from build123d import *

# Parameters (mm, degrees)
SKETCH1_W           = 240
SKETCH1_H           = 148
SKETCH1_W_2         = 235
SKETCH1_H_2         = 143
BOSS_EXTRUDE1_DEPTH = 1.2


with BuildPart() as part:
    # Sketch1 → Boss-Extrude1 (new body)
    with BuildSketch(Plane.XY):
        Rectangle(SKETCH1_W, SKETCH1_H)
        Rectangle(SKETCH1_W_2, SKETCH1_H_2, mode=Mode.SUBTRACT)
    extrude(amount=-BOSS_EXTRUDE1_DEPTH)


solid = part.part
Input: part model. Units: mm. Frame: model coordinates. Round coordinates to 2 decimals unless told otherwise and drop trailing zeros. Write each loop counter-clockwise with the first axis right and the second up, starting at its lowest first coordinate (ties: lowest second). Pieces come first, ordered by that corner, then holes.
1) Cut plane C-C (x = -67.5). Return the cut outline in (y, z).
2) Ray query, L1, parallel to X at y = -55, z = -0.55; L2, parallel to Y at x = 19, z = -0.2. Return the intervals inside material, ascending.
3) Cut plane B-B (z = -0.85). Return the cut outline in (x, y).
4) Cut plane A-A (y = -10). Return the cut outline in (x, z), then the cut area to 3 significant figures.
Geometry says:
1. outline: (-74, -1.2) - (-71.5, -1.2) - (-71.5, 0) - (-74, 0) - close; (71.5, -1.2) - (74, -1.2) - (74, 0) - (71.5, 0) - close
2. L1: x = -120 to -117.5, 117.5 to 120
2. L2: y = -74 to -71.5, 71.5 to 74
3. outline: (-120, -74) - (120, -74) - (120, 74) - (-120, 74) - close; hole (-117.5, -71.5) - (117.5, -71.5) - (117.5, 71.5) - (-117.5, 71.5) - close
4. outline: (-120, -1.2) - (-117.5, -1.2) - (-117.5, 0) - (-120, 0) - close; (117.5, -1.2) - (120, -1.2) - (120, 0) - (117.5, 0) - close
4. area: 6.00 mm2
